Drawing for the job (mm, zero at the part's lowest x, y, z). A direction names the side the tool comes from. Coordinates: 2 decimals unless noted, no trailing zeros. Loops run counter-clockwise (first coordinate to the right, second up) from the corner with the lowest first, then second, coordinate; pieces in that order, holes last. Notation, with made-up numbers: (5, -29) - (37, -29) arc R16 ccw to (37, -12) - close; hole circle Ø7 at (79.25, 1.25). An arc over 180 degrees is marked (long way). One line per item, written item: value.
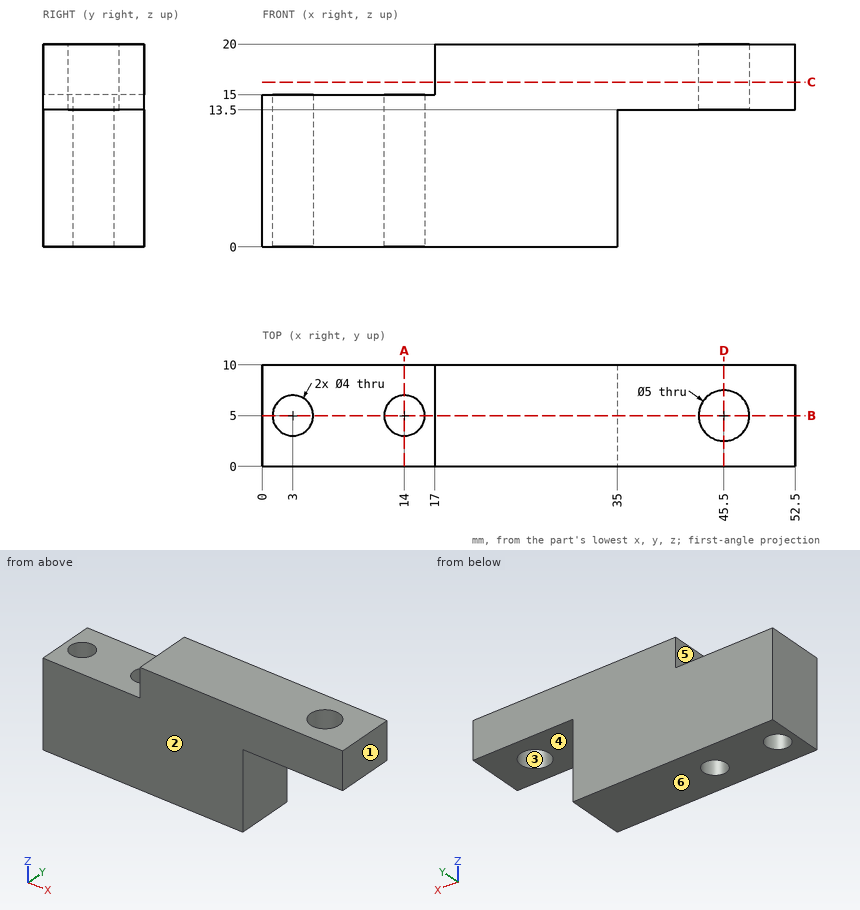
Item 1: Drop flat-ended pins along their axis: P1, Ø1.5, axis at y = 5, z = 17.5, coming from the -X side; P2, Ø6, axis at y = 6.5, z = 6.5, coming from the +X side; P3, Ø4, axis at x = 45.5, y = 5, coming from the +Z side. Give the stop position or say it passes through.
Check result:
P1: stops at x = 17
P2: stops at x = 35
P3: passes through
Item 2: Probe probe 1 along Y at (x, z) = (14, 4.25); probe 2 along Y at (x, z) = (45.5, 17.25); probe 3 along X at (y, z) = (4, 9.5). List the from-to ranges inside material, lowest first. Write a range as from..to.
Check result:
probe 1: y = 0..3, 7..10
probe 2: y = 0..2.5, 7.5..10
probe 3: x = 0..1.27, 4.73..12.27, 15.73..35
Item 3: Cut at B-B, the plane y = 5. Write the cut outline in (x, z), then the cut area to 3 significant figures.
Check result:
outline: (0, 0) - (1, 0) - (1, 15) - (0, 15) - close; (5, 0) - (12, 0) - (12, 15) - (5, 15) - close; (16, 0) - (35, 0) - (35, 13.5) - (43, 13.5) - (43, 20) - (17, 20) - (17, 15) - (16, 15) - close; (48, 13.5) - (52.5, 13.5) - (52.5, 20) - (48, 20) - close
area: 576 mm^2
Item 4: Cut at C-C, the plane z = 16.25. Write the cut outline in (x, y).
Check result:
outline: (17, 0) - (52.5, 0) - (52.5, 10) - (17, 10) - close; hole circle Ø5 at (45.5, 5)
Item 5: Cut at D-D, the plane x = 45.5. Write the cut outline in (y, z).
Check result:
outline: (0, 13.5) - (2.5, 13.5) - (2.5, 20) - (0, 20) - close; (7.5, 13.5) - (10, 13.5) - (10, 20) - (7.5, 20) - close
Item 6: Tool access for the marked faces 4, 5 and 6: list every direction of +Z, -Z, +X, -X, +Y, -Y with a clear straight run to the whole face (end or side of a thin tool).
Check result:
face 4: -Z, +X, +Y, -Y
face 5: +Z, -X, +Y, -Y
face 6: -Z, +X, -X, +Y, -Y
Item 7: Cut at A-A, the plane x = 14. Write the cut outline in (y, z).
Check result:
outline: (0, 0) - (3, 0) - (3, 15) - (0, 15) - close; (7, 0) - (10, 0) - (10, 15) - (7, 15) - close
Item 8: Pull direction Y, two halves, no side cores. Call the marked faces 1, 2 and 3: released by +Y, released by -Y, zero draft, split by the parting line, or undercut.
Check result:
face 1: zero draft
face 2: released by -Y
face 3: undercut
